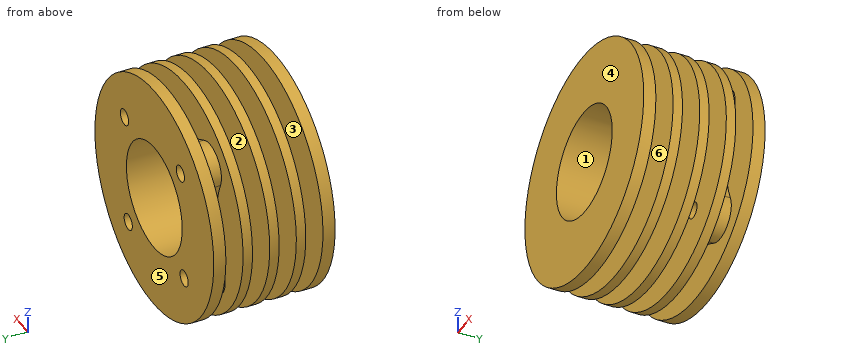
```python
from build123d import *

# Parameters (mm, degrees)
SKETCH1_R                        = 30.48
SKETCH1_R_2                      = 14.3129
BOSS_EXTRUDE1_DEPTH              = 31.75
SKETCH2_W                        = 13.97
SKETCH2_H                        = 4.5
BOSS_EXTRUDE2_START              = -7.675
BOSS_EXTRUDE2_OUTLINE_R          = 16.51
BOSS_EXTRUDE2_DEPTH              = 4.5
CUT_EXTRUDE2_REACH               = 55.536
CUT_EXTRUDE2_END_RADIUS          = 16.51
SKETCH8_R                        = 2
CUT_EXTRUDE3_REACH               = 55.536
CUT_EXTRUDE3_END_RADIUS          = 16.51
SKETCH9_R                        = 2
SKETCH10_R                       = 1
CUT_EXTRUDE4_DEPTH               = 10.141666667
TAP_DRILL_FOR_M5X0_8_TAP1_REACH  = 72.9
TAP_DRILL_FOR_M5X0_8_TAP1_BORE_R = 2.1


with BuildPart() as part:
    # Sketch1 → Boss-Extrude1 (new body)
    with BuildSketch(Plane(origin=(0, 0, 0), x_dir=(1, 0, 0), z_dir=(0, 1, 0))):
        with Locations(Location((0, 0, 0), (0, 0, 270))):
            Circle(SKETCH1_R)
        with Locations(Location((0, 0, 0), (0, 0, 270))):
            Circle(SKETCH1_R_2, mode=Mode.SUBTRACT)
    extrude(amount=BOSS_EXTRUDE1_DEPTH)

    # Sketch2 → Cut-Revolve2 (revolve, cut)
    with BuildSketch(Plane.XY, mode=Mode.PRIVATE) as cut_revolve2_sk:
        with Locations((23.495, 26.325)):
            Rectangle(SKETCH2_W, SKETCH2_H)
        with Locations((23.495, 12.391666667)):
            Rectangle(SKETCH2_W, SKETCH2_H)
        with Locations((23.495, 5.425)):
            Rectangle(SKETCH2_W, SKETCH2_H)
        with Locations((23.495, 19.358333333)):
            Rectangle(SKETCH2_W, SKETCH2_H)
    revolve(cut_revolve2_sk.sketch.rotate(Axis((0, 0, 0), (0, 1, 0)), 90), axis=Axis((0, 0, 0), (0, 1, 0)), mode=Mode.SUBTRACT)

    # Boss-Extrude2: read off the stored shape, not the designer's step
    # Boss-Extrude2 outline → Boss-Extrude2 (add)
    with BuildSketch(Plane(origin=(0, 31.75, 0), x_dir=(1, 0, 0), z_dir=(0, 1, 0)).offset(BOSS_EXTRUDE2_START)):
        with BuildLine():
            ThreePointArc((-20.446529483, 10.269067687), (-16.857865235, -1.135728529), (-18.884341927, -12.918821503))
            ThreePointArc((-18.884341927, -12.918821503), (-17.322622903, -19.825310342), (-10.269067687, -20.446529483))
            ThreePointArc((-10.269067687, -20.446529483), (1.135728529, -16.857865235), (12.918821503, -18.884341927))
            ThreePointArc((12.918821503, -18.884341927), (19.825310342, -17.322622903), (20.446529483, -10.269067687))
            ThreePointArc((20.446529483, -10.269067687), (16.857865235, 1.135728529), (18.884341927, 12.918821503))
            ThreePointArc((18.884341927, 12.918821503), (17.322622903, 19.825310342), (10.269067687, 20.446529483))
            ThreePointArc((10.269067687, 20.446529483), (-1.135728529, 16.857865235), (-12.918821503, 18.884341927))
            ThreePointArc((-12.918821503, 18.884341927), (-19.825310342, 17.322622903), (-20.446529483, 10.269067687))
        make_face()
        Circle(BOSS_EXTRUDE2_OUTLINE_R, mode=Mode.SUBTRACT)
    extrude(amount=BOSS_EXTRUDE2_DEPTH)

    # Cut-Extrude2: up to this cylinder (the profile starts inside it)
    cut_extrude2_end = Plane(origin=(0, 19.358333, 0), z_dir=(0, -1, 0)) * Cylinder(CUT_EXTRUDE2_END_RADIUS, 145.092, mode=Mode.PRIVATE)
    # Sketch8 → Cut-Extrude2 (cut, up to the surface)
    with BuildSketch(Plane.XY, mode=Mode.PRIVATE) as cut_extrude2_sk1:
        with Locations(Location((0, 19.358333333, 0), (0, 0, 180))):
            Circle(SKETCH8_R)
    cut_extrude2_tool1 = extrude(cut_extrude2_sk1.sketch, amount=CUT_EXTRUDE2_REACH, mode=Mode.PRIVATE) & cut_extrude2_end
    add(cut_extrude2_tool1.solids().sort_by_distance((0, 19.358333, 0))[0], mode=Mode.SUBTRACT)

    # Cut-Extrude3: up to this cylinder (the profile starts inside it)
    cut_extrude3_end = Plane(origin=(0, 19.358333, 0), z_dir=(0, -1, 0)) * Cylinder(CUT_EXTRUDE3_END_RADIUS, 145.092, mode=Mode.PRIVATE)
    # Sketch9 → Cut-Extrude3 (cut, up to the surface)
    with BuildSketch(Plane(origin=(0, 0, 0), x_dir=(0, 0, -1), z_dir=(1, 0, 0)), mode=Mode.PRIVATE) as cut_extrude3_sk1:
        with Locations((0, 19.358333333)):
            Circle(SKETCH9_R)
    cut_extrude3_tool1 = extrude(cut_extrude3_sk1.sketch, amount=-CUT_EXTRUDE3_REACH, mode=Mode.PRIVATE) & cut_extrude3_end
    add(cut_extrude3_tool1.solids().sort_by_distance((0, 19.358333, 0))[0], mode=Mode.SUBTRACT)

    # Sketch10 → Cut-Extrude4 (cut)
    with BuildSketch(Plane(origin=(0, 31.75, 0), x_dir=(1, 0, 0), z_dir=(0, 1, 0))):
        with Locations(Location((15.301734948, -13.370090036, 0), (0, 0, 270))):
            Circle(SKETCH10_R)
        with Locations(Location((13.370090036, 15.301734948, 0), (0, 0, 270))):
            Circle(SKETCH10_R)
        with Locations(Location((-15.301734948, 13.370090036, 0), (0, 0, 270))):
            Circle(SKETCH10_R)
        with Locations(Location((-13.370090036, -15.301734948, 0), (0, 0, 270))):
            Circle(SKETCH10_R)
    extrude(amount=-CUT_EXTRUDE4_DEPTH, mode=Mode.SUBTRACT)

    # Tap Drill for M5x0.8 Tap1 bore (on position points) → Tap Drill for M5x0.8 Tap1 (cut, up to next)
    with BuildSketch(Plane(origin=(15.301734948, 31.75, 13.370090036), x_dir=(0, 0, 1), z_dir=(0, 1, 0)), mode=Mode.PRIVATE) as tap_drill_for_m5x0_8_tap1_sk1:
        Circle(TAP_DRILL_FOR_M5X0_8_TAP1_BORE_R)
    tap_drill_for_m5x0_8_tap1_tool1 = extrude(tap_drill_for_m5x0_8_tap1_sk1.sketch, amount=-TAP_DRILL_FOR_M5X0_8_TAP1_REACH, mode=Mode.PRIVATE) & part.part
    # Tap Drill for M5x0.8 Tap1 bore (on position points) → Tap Drill for M5x0.8 Tap1 (cut, up to next)
    with BuildSketch(Plane(origin=(15.301734948, 31.75, 13.370090036), x_dir=(0, 0, 1), z_dir=(0, 1, 0)), mode=Mode.PRIVATE) as tap_drill_for_m5x0_8_tap1_sk2:
        with Locations((1.931644912, -28.671824984)):
            Circle(TAP_DRILL_FOR_M5X0_8_TAP1_BORE_R)
    tap_drill_for_m5x0_8_tap1_tool2 = extrude(tap_drill_for_m5x0_8_tap1_sk2.sketch, amount=-TAP_DRILL_FOR_M5X0_8_TAP1_REACH, mode=Mode.PRIVATE) & part.part
    # Tap Drill for M5x0.8 Tap1 bore (on position points) → Tap Drill for M5x0.8 Tap1 (cut, up to next)
    with BuildSketch(Plane(origin=(15.301734948, 31.75, 13.370090036), x_dir=(0, 0, 1), z_dir=(0, 1, 0)), mode=Mode.PRIVATE) as tap_drill_for_m5x0_8_tap1_sk3:
        with Locations((-26.740180072, -30.603469896)):
            Circle(TAP_DRILL_FOR_M5X0_8_TAP1_BORE_R)
    tap_drill_for_m5x0_8_tap1_tool3 = extrude(tap_drill_for_m5x0_8_tap1_sk3.sketch, amount=-TAP_DRILL_FOR_M5X0_8_TAP1_REACH, mode=Mode.PRIVATE) & part.part
    # Tap Drill for M5x0.8 Tap1 bore (on position points) → Tap Drill for M5x0.8 Tap1 (cut, up to next)
    with BuildSketch(Plane(origin=(15.301734948, 31.75, 13.370090036), x_dir=(0, 0, 1), z_dir=(0, 1, 0)), mode=Mode.PRIVATE) as tap_drill_for_m5x0_8_tap1_sk4:
        with Locations((-28.671824984, -1.931644912)):
            Circle(TAP_DRILL_FOR_M5X0_8_TAP1_BORE_R)
    tap_drill_for_m5x0_8_tap1_tool4 = extrude(tap_drill_for_m5x0_8_tap1_sk4.sketch, amount=-TAP_DRILL_FOR_M5X0_8_TAP1_REACH, mode=Mode.PRIVATE) & part.part
    add(tap_drill_for_m5x0_8_tap1_tool1.solids().sort_by_distance((15.301735, 31.75, 13.37009))[0], mode=Mode.SUBTRACT)
    add(tap_drill_for_m5x0_8_tap1_tool2.solids().sort_by_distance((-13.37009, 31.75, 15.301735))[0], mode=Mode.SUBTRACT)
    add(tap_drill_for_m5x0_8_tap1_tool3.solids().sort_by_distance((-15.301735, 31.75, -13.37009))[0], mode=Mode.SUBTRACT)
    add(tap_drill_for_m5x0_8_tap1_tool4.solids().sort_by_distance((13.37009, 31.75, -15.301735))[0], mode=Mode.SUBTRACT)


solid = part.part
```
CAD build for the part. Positions are in the model's coordinates, mm. Face numbers are marked on the shaded views. A direction names the side the tool comes from. Round coordinates to 2 decimals unless told otherwise and drop trailing zeros. Loops run counter-clockwise (first coordinate to the right, second up) from the corner with the lowest first, then second, coordinate; pieces in that order, holes last. Notation, with made-up numbers: M -21.75,52.5 L 23.25,52.5 A17 cw 23.25,58.5 Z; hole C -28,19.25 d8. An arc over 180 degrees is marked long. Use a Markdown table: item, result. Add a question column.
(1) Which spindle directions (+Z, -Z, +X, -X, +Y, -Y) get a long thin tool onto all of the face, cutting with end or side? Do the marked faces 1 and 2. Say none if no direction does.
(2) Cut at C-C (x = 0). State how many separate pieces and enclosed holes the cut face has, and give its area (3 significant figures).
(3) Flat gauge pins, fed straight in: pin 1 (3.5 mm diameter, centred on x = -13.37, z = 15.3, fed in from +Y); pin 2 (3 mm diameter, centred on y = 19.36, z = 0, fed in from -X); pin 3 (2 mm diameter, centred on y = 12, z = 14.5, fed in from -X). Where does each tip first touch, or does it go through?
(4) Cut at A-A (z = 25). Give the cut face in (x, y) (3 decimals), and give its area (3 significant figures).
(5) Cut at B-B (y = 27.5). Give the cut face in (x, z).
(6) Pull direction Y, two halves, no side cores. Call the marked faces 3, 4, 5 and 6: +Y half, -Y half, draft (parallel to the pull), parting line (faces both ways), or undercut.
(7) Drill centre lines: line 1 (Y direction, x = -21, z = 13) (3 decimals); line 2 (Y direction, x = 0, z = 15.35); line 3 (Z direction, x = 0.5, y = 23.5). Where is each one in solid material? Low to high.
Geometry says:
| question | item | result |
|---|---|---|
| 1 | face 1 | +Y, -Y |
| 1 | face 2 | none |
| 2 | separate pieces | 3 |
| 2 | enclosed holes | 0 |
| 2 | area | 519 mm² |
| 3 | pin 1 | stops at y = 17.11 |
| 3 | pin 2 | stops at x = 14.23 |
| 3 | pin 3 | stops at x = -9.5 |
| 4 | outline | M -17.436,0 L 17.436,0 L 17.436,3.175 L -17.436,3.175 Z; M -17.436,7.675 L 17.436,7.675 L 17.436,10.142 L -17.436,10.142 Z; M -17.436,14.642 L 17.436,14.642 L 17.436,17.108 L -17.436,17.108 Z; M -17.436,21.608 L 17.436,21.608 L 17.436,24.075 L -17.436,24.075 Z; M -17.436,28.575 L 17.436,28.575 L 17.436,31.75 L -17.436,31.75 Z |
| 4 | area | 480 mm² |
| 5 | outline | M -20.45,-10.27 A6.01 ccw -12.92,-18.88 A25.4 cw 10.27,-20.45 A6.01 ccw 18.88,-12.92 A25.4 cw 20.45,10.27 A6.01 ccw 12.92,18.88 A25.4 cw -10.27,20.45 A6.01 ccw -18.88,12.92 A25.4 cw Z; hole C -15.3,-13.37 d4.2; hole C -13.37,15.3 d4.2; hole C 0,0 d28.63; hole C 13.37,-15.3 d4.2; hole C 15.3,13.37 d4.2 |
| 6 | face 3 | undercut |
| 6 | face 4 | -Y half |
| 6 | face 5 | +Y half |
| 6 | face 6 | undercut |
| 7 | line 1 | y = 0 to 3.175, 7.675 to 10.142, 14.642 to 17.108, 21.608 to 24.075, 28.575 to 31.75 |
| 7 | line 2 | y = 0 to 17.36, 21.36 to 31.75 |
| 7 | line 3 | z = -30.48 to -14.3, 14.3 to 30.48 |
